from build123d import *

# Parameters (mm, degrees)
SKETCH1_R           = 1.5
SKETCH1_R_2         = 2.625
BOSS_EXTRUDE1_DEPTH = 3.05
FILLET2_R           = 1.6
FILLET3_R           = 2.5
FILLET4_R           = 30
FILLET5_R           = 1
FILLET6_R           = 0.75


with BuildPart() as part:
    # Sketch1 → Boss-Extrude1 (new body)
    with BuildSketch(Plane.XY):
        with BuildLine():
            Line((-5.172936369, 13.742966599), (0, 0))
            Line((0, 0), (11, 0))
            Line((11, 0), (11, 6.303908615))
            Line((11, 6.303908615), (-1.02081528, 18.324723896))
            Line((-1.02081528, 18.324723896), (-6.124201376, 31.882915925))
            ThreePointArc((-6.124201376, 31.882915925), (-6.290762776, 39.054617678), (-13.40685584, 39.961407754))
            Line((-13.40685584, 39.961407754), (-16.302263716, 42.337468617))
            Line((-16.302263716, 42.337468617), (-18.363969834, 39.82512551))
            Line((-18.363969834, 39.82512551), (-15.468561957, 37.449064647))
            ThreePointArc((-15.468561957, 37.449064647), (-15.176038376, 32.687133516), (-11.271628404, 29.945393026))
            Line((-11.271628404, 29.945393026), (-6.960865313, 18.492966599))
            Line((-6.960865313, 18.492966599), (-5.172936369, 18.492966599))
            Line((-5.172936369, 18.492966599), (-5.172936369, 13.742966599))
        make_face()
        with Locations((2.5, 3.5)):
            Circle(SKETCH1_R, mode=Mode.SUBTRACT)
        Polygon((9.727207794, 5.692209589), (7.517499103, 3.482500897), (7.464466094, 3.429467889), (1.701545827, 9.192388155), (3.964287527, 11.455129855), align=None, mode=Mode.SUBTRACT)
        Polygon((-5.650354628, 23.527354521), (-7.587877527, 28.67478155), (-6.184033792, 29.203196886), (-4.246510893, 24.055769857), align=None, mode=Mode.SUBTRACT)
        with Locations((-10.375858941, 35.371957047)):
            Circle(SKETCH1_R_2, mode=Mode.SUBTRACT)
    extrude(amount=BOSS_EXTRUDE1_DEPTH)

    # Sketch3 → CSK for M3 Flat Head Machine Screw1 (revolve, cut)
    with BuildSketch(Plane(origin=(2.5, 3.5, 3.05), x_dir=(0, -1, 0), z_dir=(1, 0, 0))):
        Polygon((0, 0), (0, 3.05), (1.55, 3.05), (1.55, 1.6), (3.15, 0), align=None)
    revolve(axis=Axis((2.5, 3.5, 9.4), (0, 0, -1)), mode=Mode.SUBTRACT)

    # Fillet2
    fillet2_edges = [part.edges().sort_by_distance(p)[0] for p in [
        (-5.172936369, 18.492966599, 1.525),
    ]]
    fillet(fillet2_edges, radius=FILLET2_R)

    # Fillet3
    fillet3_edges = [part.edges().sort_by_distance(p)[0] for p in [
        (-6.124201376, 31.882915925, 1.525),
        (-11.271628404, 29.945393026, 1.525),
        (-15.468561957, 37.449064647, 1.525),
        (-13.40685584, 39.961407754, 1.525),
    ]]
    fillet(fillet3_edges, radius=FILLET3_R)

    # Fillet4
    fillet4_edges = [part.edges().sort_by_distance(p)[0] for p in [
        (-1.02081528, 18.324723896, 1.525),
    ]]
    fillet(fillet4_edges, radius=FILLET4_R)

    # Fillet5
    fillet5_edges = [part.edges().sort_by_distance(p)[0] for p in [
        (-6.960865313, 18.492966599, 1.525),
        (-5.172936369, 13.742966599, 1.525),
    ]]
    fillet(fillet5_edges, radius=FILLET5_R)

    # Fillet6
    fillet6_edges = [part.edges().sort_by_distance(p)[0] for p in [
        (-4.246510893, 24.055769857, 1.525),
        (-5.650354628, 23.527354521, 1.525),
        (-6.184033792, 29.203196886, 1.525),
        (-7.587877527, 28.67478155, 1.525),
    ]]
    fillet(fillet6_edges, radius=FILLET6_R - 0.0001)  # a hair under: the kernel refuses the full size


solid = part.part
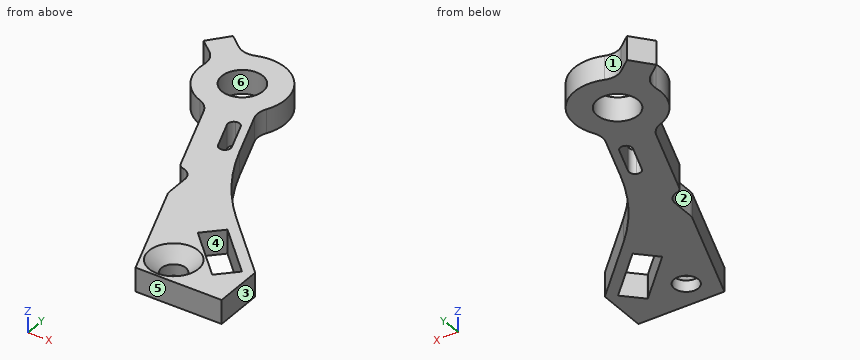
Geometry check sheet. Reference: the model listing, model coordinates, mm. Face numbers are marked on the shaded views. A direction names the side the tool comes from. Round coordinates to 2 decimals unless told otherwise and drop trailing zeros. Loops run counter-clockwise (first coordinate to the right, second up) from the corner with the lowest first, then second, coordinate; pieces in that order, holes last.
Item 1: Thickness scan on line 1 (Y direction, x = 3.5, z = 0.7); line 2 (Y direction, x = 2.5, z = 0.4); line 3 (X direction, y = 24, z = 0.95). Record the ranges inside material, lowest first.
Item 2: Cross-section at C-C on y = 16. Record the boundary of the cut face in (x, z).
Item 3: Cross-section at D-D on x = -2.5. Record the boundary of the cut face in (y, z), then the cut area to 3 significant figures.
Item 4: Mould release check, pull along Y, two halves, no side actions. Record for the marked faces 3, 4, 5 and 6: pulls with the +Y half, pulls with the -Y half, needs draft (parallel to the pull), parting line crosses it, or undercut.
Item 5: Gauge pin test, flat end, axial feed: pin 1 (4 mm diameter, centred on x = 2.5, y = 3.5, fed in from +Z). Record the tip position at first contact, or that the pin passes through.
Item 6: Cross-section at A-A on x = 2.5. Record the boundary of the cut face in (y, z).
Item 7: Cross-section at B-B on z = 2.1. Count the separate pieces of the cut face and the enclosed holes in it, then the cut area to 3 significant figures.
Item 8: Access from +Z, -Z, +X, -X, +Y, -Y to the whole of each face (thin tool, end or side, straight path). Record for the marked faces 1 and 2.
Answer sheet:
1. line 1: y = 0 to 2.32, 4.68 to 7.39, 10.99 to 13.8
1. line 2: y = 0 to 1.95, 5.05 to 8.39, 9.99 to 14.86
1. line 3: x = -9.03 to -5.78, -4.65 to -3.15
2. outline: (-5.17, 0) - (1.52, 0) - (1.52, 3.05) - (-5.17, 3.05) - close
3. outline: (6.64, 0) - (22.46, 0) - (22.46, 3.05) - (6.64, 3.05) - close
3. area: 48.2 mm2
4. face 3: needs draft
4. face 4: undercut
4. face 5: pulls with the -Y half
4. face 6: undercut
5. pin 1: stops at z = 1.9
6. outline: (0, 0) - (1.95, 0) - (1.95, 1.45) - (0.35, 3.05) - (0, 3.05) - close; (5.05, 0) - (8.39, 0) - (8.39, 3.05) - (6.65, 3.05) - (5.05, 1.45) - close; (9.99, 0) - (14.86, 0) - (14.86, 3.05) - (9.99, 3.05) - close
7. separate pieces: 1
7. enclosed holes: 4
7. area: 300 mm2
8. face 1: +Z, -Z, +Y
8. face 2: +Z, -Z, -X, -Y
